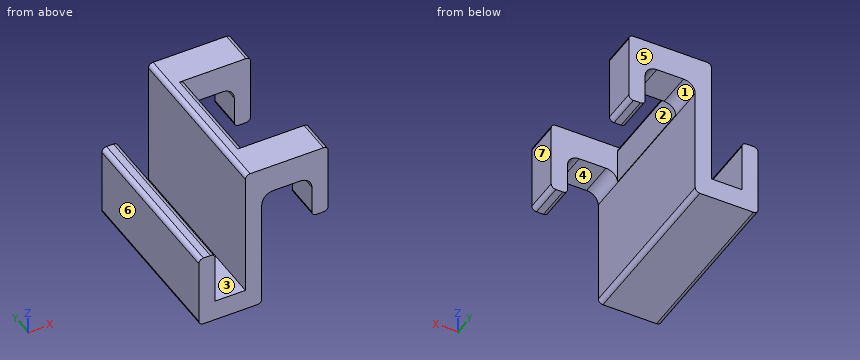
Autodesk Fusion 360 part; units mm, degrees
sketch "Sketch1" plane through (0, 0, 0) normal (0, 1, 0) x (1, 0, 0)
  line L0 (-10.8509, -30.1905) -> (-10.8509, -7.1905)
  line L1 (-10.8509, -7.1905) -> (2.1491, -7.1905)
  line L2 (2.1491, -7.1905) -> (2.1491, -63.1905)
  line L3 (2.1491, -63.1905) -> (9.1491, -63.1905)
  line L4 (9.1491, -63.1905) -> (9.1491, 1.8095)
  line L5 (9.1491, 1.8095) -> (-17.8509, 1.8095)
  line L6 (-17.8509, 1.8095) -> (-17.8509, -30.1905)
  line L7 (-17.8509, -30.1905) -> (-10.8509, -30.1905)
  line L8 (9.1491, -63.1905) -> (38, -63.1905)
  line L9 (37.6491, -63.1989) -> (37.6491, -32)
  line L10 (37.6491, -32) -> (30.6491, -32)
  line L11 (30.6491, -32) -> (30.6491, -51)
  line L12 (30.6491, -51) -> (9.1491, -51)
  dimension "d11" = 65
  dimension "d15" = 27
  dimension "d16" = 7
  dimension "d17" = 13
  dimension "d18" = 23
  dimension "d24" = 35.5
  dimension "d28" = 21.5
  dimension "d29" = 7
  dimension "d37" = 32
extrude "Extrude2" add sketch "Sketch1" along normal blind 75 makes body 1
fillet "Fillet4" radius 5 2 edges at (9.1491, 37.5, 51) (30.6491, 37.5, 51) on bodies 1
box "BoxPrimitive1" add length 45 width 45 height 45 placed x (0, 0, 1) y (1, 0, 0) z (0, 1, 0) at (45, 0, 23) separate body makes body 2
move_body "Move9" bodies 2 to x (1, 0, 0) y (0, 1, 0) z (0, 0, 1) at (-35.8367, 15, -2.9383)
combine "Combine1" operation cut target body 1 tool bodies 2
fillet "Fillet5" radius 2 8 edges at (2.1491, 37.5, 63.1905) (37.6491, 7.5, 63.1905) (37.6491, 67.5, 63.1905) (9.1633, 37.5, 63.1905) (30.6491, 7.5, 32) (37.6491, 7.5, 32) (30.6491, 67.5, 32) (37.6491, 67.5, 32) on bodies 1
fillet "Fillet6" radius 2 4 edges at (-17.8509, 37.5, 30.1905) (9.1491, 37.5, -1.8095) (-17.8509, 37.5, -1.8095) (-10.8509, 37.5, 30.1905) on bodies 1
Geometry check sheet. Reference: the model listing, model coordinates, mm. Face numbers are marked on the shaded views. A direction names the side the tool comes from. Round coordinates to 2 decimals unless told otherwise and drop trailing zeros. Order: outer loops, then holes, each group sorted by start corner. A loop starts at its lowest first (then second) coordinate and runs counter-clockwise, first axis right, second up. Notation, with made-up numbers: (32, 55) - (36, 55) arc R21 ccw to (36, 71) - close; hole circle Ø10 at (-30.75, 68). An arc over 180 degrees is marked (long way). Use a Markdown table: item, result. Add a question column.
1) Mould release check, pull along X, two halves, no side actions. Record for the marked faces 4, 5, 6 and 7: released by +X, released by -X, zero draft, split by the parting line, or undercut.
2) Section check B-B (z = 25). Record the cut outline in (x, y), then the cut area to 3 significant figures.
3) Gauge pin test, flat ends, axial feed: P1, Ø14.5, axis at x = -1.5, y = 22.5, coming from the +Z side; P2, Ø6, axis at x = 22.5, y = 7.5, coming from the -Z side; P3, Ø13, axis at y = 65, z = 37.5, coming from the -X side; P4, Ø7.5, axis at y = 37.5, z = 52, coming from the +X side. Record the tip position at first contact, or that the pin passes through.
4) Section check D-D (y = 70). Record the cut outline in (x, z), then the cut area to 3 significant figures.
5) Set-up check for the marked faces 1, 2 and 3: record each of +Z, -Z, +X, -X, +Y, -Y from which the full face is reachable in a straight line by a thin tool's end or side.
6) Section check C-C (x = 15.5). Record the cut outline in (y, z), then the cut area to 3 significant figures.
7) Section check A-A (z = 45). Record the cut outline in (x, y), then the cut area to 3 significant figures.
8) Thickness scan on line 1 along X through (y, z) = (66.5, 20.5); line 2 along X through (y, z) = (67, 34.5); line 3 along Y through (x, z) = (19, 59). Record the ranges inside material, lowest first.
Established:
| question | item | result |
|---|---|---|
| 1 | face 4 | undercut |
| 1 | face 5 | zero draft |
| 1 | face 6 | released by -X |
| 1 | face 7 | released by +X |
| 2 | outline | (-17.85, 0) - (-10.85, 0) - (-10.85, 75) - (-17.85, 75) - close; (2.15, 0) - (9.15, 0) - (9.15, 75) - (2.15, 75) - close |
| 2 | area | 1,050 mm2 |
| 3 | P1 | z = 63.19 |
| 3 | P2 | z = 51 |
| 3 | P3 | x = 2.15 |
| 3 | P4 | x = 9.16 |
| 4 | outline | (-17.85, 0.19) arc R2 ccw to (-15.85, -1.81) - (7.15, -1.81) arc R2 ccw to (9.15, 0.19) - (9.15, 46) arc R5 cw to (14.15, 51) - (25.65, 51) arc R5 cw to (30.65, 46) - (30.65, 34) arc R2 ccw to (32.65, 32) - (35.65, 32) arc R2 ccw to (37.65, 34) - (37.65, 61.19) arc R2 ccw to (35.65, 63.19) - (4.15, 63.19) arc R2 ccw to (2.15, 61.19) - (2.15, 7.19) - (-10.85, 7.19) - (-10.85, 28.19) arc R2 ccw to (-12.85, 30.19) - (-15.85, 30.19) arc R2 ccw to (-17.85, 28.19) - close |
| 4 | area | 1,280 mm2 |
| 5 | face 1 | -Z, +Y, -Y |
| 5 | face 2 | +Z, -Z, +X |
| 5 | face 3 | +Z, +Y, -Y |
| 6 | outline | (0, 51) - (15, 51) - (15, 63.19) - (0, 63.19) - close; (60, 51) - (75, 51) - (75, 63.19) - (60, 63.19) - close |
| 6 | area | 366 mm2 |
| 7 | outline | (2.15, 0) - (9.15, 0) - (9.15, 75) - (2.15, 75) - close; (30.65, 0) - (37.65, 0) - (37.65, 15) - (30.65, 15) - close; (30.65, 60) - (37.65, 60) - (37.65, 75) - (30.65, 75) - close |
| 7 | area | 735 mm2 |
| 8 | line 1 | -17.85 to -10.85, 2.15 to 9.15 |
| 8 | line 2 | 2.15 to 9.15, 30.65 to 37.65 |
| 8 | line 3 | 0 to 15, 60 to 75 |
